from build123d import *

# Parameters (mm, degrees)
F_1_4_20_TAPPED_HOLE1_D     = 5.1054
F_1_4_20_TAPPED_HOLE1_DEPTH = 13.335
F_1_4_20_TAPPED_HOLE1_TIP   = 1.533816902
SKETCH4_W                   = 4.064
SKETCH4_H                   = 3.0734
CHAMFER1_SIZE               = 0.127
F_8_32_TAPPED_HOLE1_D       = 3.4544
CUT_EXTRUDE1_REACH          = 182.613
SKETCH7_W                   = 50.8
SKETCH7_H                   = 2.565921067


with BuildPart() as part:
    # Sketch1 → Revolve1 (revolve)
    with BuildSketch(Plane.XY, mode=Mode.PRIVATE) as revolve1_sk:
        Polygon((109.7915, 0), (109.7915, 2.54), (105.7783, 2.54), (99.4283, 2.54), (99.4283, 9.525), (80.3783, 9.525), (80.3783, 19.05), (105.7783, 19.05), (127, 19.05), (127, 0), align=None)
    revolve(revolve1_sk.sketch.rotate(Axis((0, 0, 0), (0, 1, 0)), 90), axis=Axis((0, 0, 0), (0, 1, 0)))

    # 1/4-20 Tapped Hole1
    with Locations(Plane(origin=(0, 19.05, 0), x_dir=(1, 0, 0), z_dir=(0, 1, 0))):
        with Locations((0, 106.045), (68.164412069, 81.235182971), (104.433938168, 18.414521001), (91.837663944, -53.0225), (36.269526099, -99.649703971), (-36.269526099, -99.649703971), (-91.837663944, -53.0225), (-104.433938168, 18.414521001), (-68.164412069, 81.235182971)):
            Hole(F_1_4_20_TAPPED_HOLE1_D / 2, depth=F_1_4_20_TAPPED_HOLE1_DEPTH)
            with Locations((0, 0, -(F_1_4_20_TAPPED_HOLE1_DEPTH + F_1_4_20_TAPPED_HOLE1_TIP / 2))):  # 118° drill point
                Cone(0, F_1_4_20_TAPPED_HOLE1_D / 2, F_1_4_20_TAPPED_HOLE1_TIP, mode=Mode.SUBTRACT)

    # Sketch4 → Cut-Revolve1 (revolve, cut)
    with BuildSketch(Plane.XY, mode=Mode.PRIVATE) as cut_revolve1_sk:
        with Locations((97.0788, 17.5133)):
            Rectangle(SKETCH4_W, SKETCH4_H)
    revolve(cut_revolve1_sk.sketch.rotate(Axis((0, 19.05, 0), (0, -1, 0)), 90), axis=Axis((0, 19.05, 0), (0, -1, 0)), mode=Mode.SUBTRACT)

    # Chamfer1
    chamfer1_edges = [part.edges().sort_by_distance(p)[0] for p in [
        (0, 19.05, -95.0468),
        (0, 19.05, -99.1108),
    ]]
    chamfer(chamfer1_edges, length=CHAMFER1_SIZE)

    # #8-32 Tapped Hole1 (through all)
    with Locations(Plane(origin=(0, 9.525, 0), x_dir=(-1, 0, 0), z_dir=(0, -1, 0))):
        with Locations((6.35, -85.09), (-6.35, -85.09)):
            Hole(F_8_32_TAPPED_HOLE1_D / 2)

    # Sketch7 → Cut-Extrude1 (cut, up to next)
    with BuildSketch(Plane(origin=(0, 19.05, 0), x_dir=(1, 0, 0), z_dir=(0, 1, 0)), mode=Mode.PRIVATE) as cut_extrude1_sk1:
        with Locations((0, -125.717039467)):
            Rectangle(SKETCH7_W, SKETCH7_H)
    cut_extrude1_tool1 = extrude(cut_extrude1_sk1.sketch, amount=-CUT_EXTRUDE1_REACH, mode=Mode.PRIVATE) & part.part
    add(cut_extrude1_tool1.solids().sort_by_distance((0, 19.05, 125.717039))[0], mode=Mode.SUBTRACT)


solid = part.part
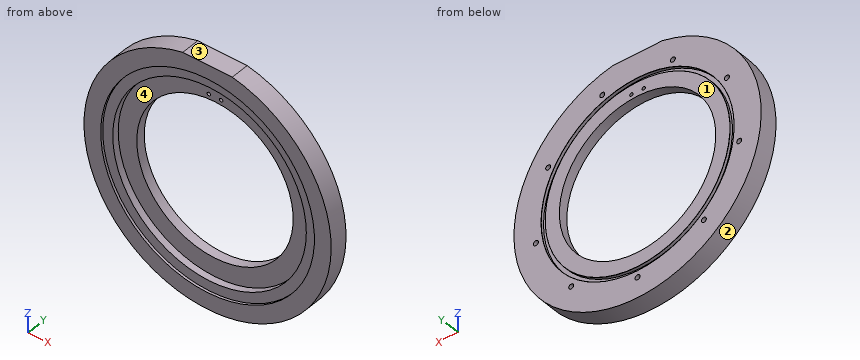
Can you work these out from the model? Positions are in its coordinate system, mm. Face numbers are marked on the shaded views. Coordinates: 2 decimals unless noted, no trailing zeros. Use one line per item in the form item = value.
Q1. Will these pins go through, and if not, where does the flat tip stop? P1, Ø5, axis at y = 16.5, z = 12, coming from the +X side; P2, Ø6, axis at x = 98, z = 37.5, coming from the -Y side; P3, Ø6, axis at x = 64, y = 12.5, coming from the -Z side; P4, Ø3, axis at x = 6.35, z = 85.09, coming from the -Y side.
From the geometry:
P1 = 126.64
P2 = 2.54
P3 = -111.39
P4 = through
Q2. We'd pull the mould along Z, two halves only. Please class the marked faces 1, 2, 3 and 4: released by +Z, released by -Z, zero draft, split by the parting line, or undercut.
From the geometry:
face_1 = zero draft
face_2 = split by the parting line
face_3 = released by +Z
face_4 = undercut
Q3. I need wall thicknesses on L1, parallel to X at y = 17.45, z = 0; L2, parallel to Z at x = -37, y = 15.25; L3, parallel to X at y = 7.75, z = -82. Which ranges of each line are inside material? Lowest first, please.
From the geometry:
L1 = -127 to -99.11, -95.05 to -80.38, 80.38 to 95.05, 99.11 to 127
L2 = -121.49 to -71.36, 71.36 to 97.2, 102.1 to 121.49
L3 = -96.98 to -70.6, -65.73 to -56.23, 56.23 to 65.73, 70.6 to 96.98
